Part model, mm, in its own coordinate system. Give positions to 0.01 mm unless a question says otherwise; leave off trailing zeros. Write each loop counter-clockwise with the first axis right and the second up, starting at its lowest first coordinate (ties: lowest second). Pieces come first, ordered by that corner, then holes. Notation, with made-up numbers: M 57.25,45.25 L 97.25,45.25 A35 ccw 97.25,79.25 Z; hole C 45.25,-21 d5. An arc over 180 degrees is marked long. Use CSV: the item, a comma, the result in double quotes. Start each with the question number.
1. Drill centre lines: line 1 along Y through (x, z) = (-0.5, 21); line 2 along X through (y, z) = (-12, 50.8); line 3 along Y through (x, z) = (-5.8, 12.7). Where is each one in solid material? Low to high. Write a range as from..to.
2. Band-saw the part on C-C, the plane z = 142.5. List the corners of the cut face in (x, y).
3. Band-saw the part on A-A, the plane x = 4. List the corners of the cut face in (y, z).
4. Band-saw the part on B-B, the plane y = -6.75. List the corners of the cut face in (x, z).
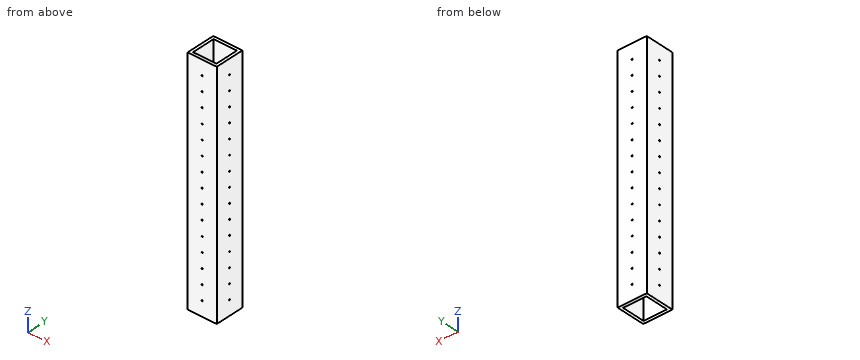
from build123d import *

# Parameters (mm, degrees)
SKETCH1_W               = 25.4
SKETCH1_H               = 25.4
SKETCH1_W_2             = 20.32
SKETCH1_H_2             = 20.32
BOSS_EXTRUDE1_DEPTH     = 203.2
SKETCH2_R               = 0.5
CUT_EXTRUDE1_DEPTH      = 1
CUT_EXTRUDE1_DEPTH_BACK = 26.4
SKETCH3_R               = 0.5
CUT_EXTRUDE2_DEPTH      = 1
CUT_EXTRUDE2_DEPTH_BACK = 26.4


with BuildPart() as part:
    # Sketch1 → Boss-Extrude1 (new body)
    with BuildSketch(Plane.XY):
        with Locations((6.158862876, -0.297324415)):
            Rectangle(SKETCH1_W, SKETCH1_H)
        with Locations((6.158862876, -0.297324415)):
            Rectangle(SKETCH1_W_2, SKETCH1_H_2, mode=Mode.SUBTRACT)
    extrude(amount=BOSS_EXTRUDE1_DEPTH)

    # Sketch2 → Cut-Extrude1 (cut, two sides)
    with BuildSketch(Plane(origin=(18.858862876, 0, 0), x_dir=(0, 0, -1), z_dir=(1, 0, 0))) as cut_extrude1_sk:
        with Locations((-190.5, -0.297324415)):
            Circle(SKETCH2_R)
        with Locations((-177.8, -0.297324415)):
            Circle(SKETCH2_R)
        with Locations((-165.1, -0.297324415)):
            Circle(SKETCH2_R)
        with Locations((-152.4, -0.297324415)):
            Circle(SKETCH2_R)
        with Locations((-139.7, -0.297324415)):
            Circle(SKETCH2_R)
        with Locations((-127, -0.297324415)):
            Circle(SKETCH2_R)
        with Locations((-114.3, -0.297324415)):
            Circle(SKETCH2_R)
        with Locations((-101.6, -0.297324415)):
            Circle(SKETCH2_R)
        with Locations((-88.9, -0.297324415)):
            Circle(SKETCH2_R)
        with Locations((-76.2, -0.297324415)):
            Circle(SKETCH2_R)
        with Locations((-63.5, -0.297324415)):
            Circle(SKETCH2_R)
        with Locations((-50.8, -0.297324415)):
            Circle(SKETCH2_R)
        with Locations((-38.1, -0.297324415)):
            Circle(SKETCH2_R)
        with Locations((-25.4, -0.297324415)):
            Circle(SKETCH2_R)
        with Locations((-12.7, -0.297324415)):
            Circle(SKETCH2_R)
    extrude(amount=CUT_EXTRUDE1_DEPTH, mode=Mode.SUBTRACT)
    extrude(cut_extrude1_sk.sketch, amount=-CUT_EXTRUDE1_DEPTH_BACK, mode=Mode.SUBTRACT)

    # Sketch3 → Cut-Extrude2 (cut, two sides)
    with BuildSketch(Plane(origin=(0, 12.402675585, 0), x_dir=(1, 0, 0), z_dir=(0, 1, 0))) as cut_extrude2_sk:
        with Locations((6.158862876, -190.5)):
            Circle(SKETCH3_R)
        with Locations((6.158862876, -177.8)):
            Circle(SKETCH3_R)
        with Locations((6.158862876, -165.1)):
            Circle(SKETCH3_R)
        with Locations((6.158862876, -152.4)):
            Circle(SKETCH3_R)
        with Locations((6.158862876, -139.7)):
            Circle(SKETCH3_R)
        with Locations((6.158862876, -127)):
            Circle(SKETCH3_R)
        with Locations((6.158862876, -114.3)):
            Circle(SKETCH3_R)
        with Locations((6.158862876, -101.6)):
            Circle(SKETCH3_R)
        with Locations((6.158862876, -88.9)):
            Circle(SKETCH3_R)
        with Locations((6.158862876, -76.2)):
            Circle(SKETCH3_R)
        with Locations((6.158862876, -63.5)):
            Circle(SKETCH3_R)
        with Locations((6.158862876, -50.8)):
            Circle(SKETCH3_R)
        with Locations((6.158862876, -38.1)):
            Circle(SKETCH3_R)
        with Locations((6.158862876, -25.4)):
            Circle(SKETCH3_R)
        with Locations((6.158862876, -12.7)):
            Circle(SKETCH3_R)
    extrude(amount=CUT_EXTRUDE2_DEPTH, mode=Mode.SUBTRACT)
    extrude(cut_extrude2_sk.sketch, amount=-CUT_EXTRUDE2_DEPTH_BACK, mode=Mode.SUBTRACT)


solid = part.part
Output:
1,line 1,"y = -13..-10.46, 9.86..12.4"
1,line 2,"x = -6.54..5.66, 6.66..18.86"
1,line 3,"y = -13..-0.8, 0.2..12.4"
2,outline,"M -6.54,-13 L 18.86,-13 L 18.86,12.4 L -6.54,12.4 Z; hole M -4,-10.46 L 16.32,-10.46 L 16.32,9.86 L -4,9.86 Z"
3,outline,"M -13,0 L -10.46,0 L -10.46,203.2 L -13,203.2 Z; M 9.86,0 L 12.4,0 L 12.4,203.2 L 9.86,203.2 Z"
4,outline,"M -6.54,0 L -4,0 L -4,203.2 L -6.54,203.2 Z; M 16.32,0 L 18.86,0 L 18.86,203.2 L 16.32,203.2 Z"
